Work out the finished part from the listing and answer in its coordinate system (mm). Give positions to 0.01 mm unless a question says otherwise; leave off trailing zeros. Loops run counter-clockwise (first coordinate to the right, second up) from the corner with the lowest first, then second, coordinate; pieces in that order, holes last. Notation, with made-up numbers: (86, 52.25) - (122, 52.25) arc R31 cw to (122, 76.25) - close; hole circle Ø1 at (2, -25). An arc over 180 degrees is marked (long way). One line per question, with ' | ' between items.
from build123d import *

# Parameters (mm, degrees)
SKETCH_1_R          = 1.575
SKETCH_1_R_2        = 14.5
EXTRUDE_1_DEPTH     = 3
CUT_EXTRUDE_START   = -3
CUT_EXTRUDE_1_DEPTH = 3
SKETCH_3_W          = 9
SKETCH_3_H          = 4
EXTRUDE_2_DEPTH     = 3
SKETCH_4_R          = 4
SKETCH_4_R_2        = 1.4
EXTRUDE_3_DEPTH     = 3
SKETCH_5_W          = 57.078231857
SKETCH_5_H          = 48.607322339
CUT_EXTRUDE_2_DEPTH = 10
SKETCH_6_W          = 9
SKETCH_6_H          = 3
EXTRUDE_4_DEPTH     = 3
FILLET_1_R          = 2
FILLET_2_R          = 3
FILLET_3_R          = 2


with BuildPart() as part:
    # 草图1 → 凸台-拉伸1 (new body)
    with BuildSketch(Plane.XY):
        with BuildLine():
            ThreePointArc((7.5, 0), (7.485279444, 0.469671844), (7.441175562, 0.9375))
            Line((7.441175562, 0.9375), (4.960783708, 20.625))
            ThreePointArc((4.960783708, 20.625), (0, 25), (-4.960783708, 20.625))
            Line((-4.960783708, 20.625), (-7.441175562, 0.9375))
            ThreePointArc((-7.441175562, 0.9375), (-7.485279444, 0.469671844), (-7.5, 0))
            Line((-7.5, 0), (-7.5, -69.31788212))
            ThreePointArc((-7.5, -69.31788212), (0, -112), (7.5, -69.31788212))
            Line((7.5, -69.31788212), (7.5, 0))
        make_face()
        with Locations((-12.374368671, -102.374368671)):
            Circle(SKETCH_1_R, mode=Mode.SUBTRACT)
        with Locations((-12.374368671, -77.625631329)):
            Circle(SKETCH_1_R, mode=Mode.SUBTRACT)
        with Locations((0, -90)):
            Circle(SKETCH_1_R_2, mode=Mode.SUBTRACT)
        with Locations((12.374368671, -102.374368671)):
            Circle(SKETCH_1_R, mode=Mode.SUBTRACT)
        with Locations((12.374368671, -77.625631329)):
            Circle(SKETCH_1_R, mode=Mode.SUBTRACT)
        Circle(SKETCH_1_R, mode=Mode.SUBTRACT)
        with Locations((0, 20)):
            Circle(SKETCH_1_R, mode=Mode.SUBTRACT)
    extrude(amount=EXTRUDE_1_DEPTH)

    # 草图2 → 切除-拉伸1 (cut)
    with BuildSketch(Plane.XY.offset(3).offset(CUT_EXTRUDE_START)):
        with BuildLine():
            Line((0, -68), (0, -5))
            ThreePointArc((0, -5), (-2.655442773, -4.236581603), (-4.5, -2.179449472))
            Line((-4.5, -2.179449472), (-4.5, -68.465144533))
            ThreePointArc((-4.5, -68.465144533), (-2.261988032, -68.116595097), (0, -68))
        make_face()
        with BuildLine():
            ThreePointArc((4.5, -2.179449472), (2.655442773, -4.236581603), (0, -5))
            Line((0, -5), (0, -68))
            ThreePointArc((0, -68), (2.261988032, -68.116595097), (4.5, -68.465144533))
            Line((4.5, -68.465144533), (4.5, -2.179449472))
        make_face()
        with BuildLine():
            Line((-2.557135445, 15.70336663), (-4.192274153, 2.724855487))
            ThreePointArc((-4.192274153, 2.724855487), (0, 5), (4.192274153, 2.724855487))
            Line((4.192274153, 2.724855487), (2.557135445, 15.70336663))
            ThreePointArc((2.557135445, 15.70336663), (0, 15), (-2.557135445, 15.70336663))
        make_face()
    extrude(amount=CUT_EXTRUDE_1_DEPTH, mode=Mode.SUBTRACT)

    # 草图3 → 凸台-拉伸2 (add)
    with BuildSketch(Plane.XY.offset(3)):
        with Locations((0, -45)):
            Rectangle(SKETCH_3_W, SKETCH_3_H)
        with Locations((0, -25)):
            Rectangle(SKETCH_3_W, SKETCH_3_H)
    extrude(amount=-EXTRUDE_2_DEPTH)

    # 草图4 → 凸台-拉伸3 (add)
    # profile 1 of 2: a face of its own
    with BuildSketch(Plane.XY.offset(3)):
        with Locations((-9, -61.2)):
            Circle(SKETCH_4_R)
        with Locations((-9, -61.2)):
            Circle(SKETCH_4_R_2, mode=Mode.SUBTRACT)
    # profile 2 of 2: a face of its own
    with BuildSketch(Plane.XY.offset(3)):
        with Locations((9, -61.2)):
            Circle(SKETCH_4_R)
        with Locations((9, -61.2)):
            Circle(SKETCH_4_R_2, mode=Mode.SUBTRACT)
    extrude(amount=-EXTRUDE_3_DEPTH)

    # 草图5 → 切除-拉伸2 (cut)
    with BuildSketch(Plane.XY.offset(3)):
        with Locations((3.178219729, -91.30366117)):
            Rectangle(SKETCH_5_W, SKETCH_5_H)
    extrude(amount=-CUT_EXTRUDE_2_DEPTH, mode=Mode.SUBTRACT)

    # 草图6 → 凸台-拉伸4 (add)
    with BuildSketch(Plane.XY.offset(3)):
        with Locations((0, -65.5)):
            Rectangle(SKETCH_6_W, SKETCH_6_H)
    extrude(amount=-EXTRUDE_4_DEPTH)

    # 圆角1
    fillet_1_edges = [part.edges().sort_by_distance(p)[0] for p in [
        (-4.5, -27, 1.5),
        (-4.5, -23, 1.5),
        (4.5, -23, 1.5),
        (4.5, -27, 1.5),
        (-2.557135445, 15.70336663, 1.5),
        (2.557135445, 15.70336663, 1.5),
        (4.192274153, 2.724855487, 1.5),
        (-4.192274153, 2.724855487, 1.5),
        (-4.5, -2.179449472, 1.5),
        (4.5, -2.179449472, 1.5),
        (-4.5, -47, 1.5),
        (-4.5, -43, 1.5),
        (4.5, -43, 1.5),
        (4.5, -47, 1.5),
    ]]
    fillet(fillet_1_edges, radius=FILLET_1_R)

    # 圆角2
    # the kernel refuses this fillet: 3 mm, written as the material it adds along each edge
    with BuildSketch(Plane(origin=(-7.5, -64.908099244, 0), x_dir=(0, -1, 0), z_dir=(0, 0, 1))) as fillet_2_piece_1:
        with BuildLine():
            CenterArc((3.170220896, -2.799504541), FILLET_2_R, 111.06581136, 58.235536144)
            Line((0.222369408, -2.242574024), (0.163412378, -2.231435413))
            ThreePointArc((0.163412378, -2.231435413), (0.21267274, -1.11122365), (-0.055621489, -0.0225))
            Line((-0.055621489, -0.0225), (0, 0.06))
            ThreePointArc((0, 0.06), (1.045950378, 0.06), (2.070334354, 0.055990091))
            Line((2.070334354, 0.055990091), (2.091900756, 0))
        make_face()
    extrude(amount=3)
    with BuildSketch(Plane(origin=(-7.5, -57.491900756, 0), x_dir=(0, 1, 0), z_dir=(0, 0, 1))) as fillet_2_piece_2:
        with BuildLine():
            CenterArc((3.129297922, 3), FILLET_2_R, 192.373625116, 77.626374884)
            Line((0.198984851, 2.357142857), (0.14037859, 2.344285714))
            ThreePointArc((0.14037859, 2.344285714), (0.217936404, 1.168572647), (-0.055621489, 0.0225))
            Line((-0.055621489, 0.0225), (0, -0.06))
            Line((0, -0.06), (3.129297922, -0.06))
            Line((3.129297922, -0.06), (3.129297922, 0))
        make_face()
    extrude(amount=3)
    with BuildSketch(Plane(origin=(7.5, -64.908099244, 0), x_dir=(0, -1, 0), z_dir=(0, 0, 1))) as fillet_2_piece_3:
        with BuildLine():
            CenterArc((3.170220896, 2.799504541), FILLET_2_R, 190.698652496, 58.235536144)
            Line((0.222369408, 2.242574024), (0.163412378, 2.231435413))
            ThreePointArc((0.163412378, 2.231435413), (0.21267274, 1.11122365), (-0.055621489, 0.0225))
            Line((-0.055621489, 0.0225), (0, -0.06))
            ThreePointArc((0, -0.06), (1.045950378, -0.06), (2.070334354, -0.055990091))
            Line((2.070334354, -0.055990091), (2.091900756, 0))
        make_face()
    extrude(amount=3)
    with BuildSketch(Plane(origin=(7.5, -57.491900756, 0), x_dir=(0.996455748224994, 0.08411861761445558, 0), z_dir=(0, 0, 1))) as fillet_2_piece_4:
        with BuildLine():
            CenterArc((3.25259946, 2.865851049), FILLET_2_R, 175.17465614, 77.626374884)
            Line((0.263232215, 3.118206902), (0.20344487, 3.123254019))
            Line((0.20344487, 3.123254019), (-0.059787345, 0.005047117))
            Line((-0.059787345, 0.005047117), (0.017741452, -0.057317021))
            ThreePointArc((0.017741452, -0.057317021), (1.18276344, 0.118865267), (2.347785428, -0.057317021))
            Line((2.347785428, -0.057317021), (2.36552688, 0))
        make_face()
    extrude(amount=3)

    # 圆角3
    fillet_3_edges = [part.edges().sort_by_distance(p)[0] for p in [
        (-7.5, -67, 1.5),
        (7.5, -67, 1.5),
        (-4.5, -64, 1.5),
        (4.5, -64, 1.5),
    ]]
    fillet(fillet_3_edges, radius=FILLET_3_R)


solid = part.part
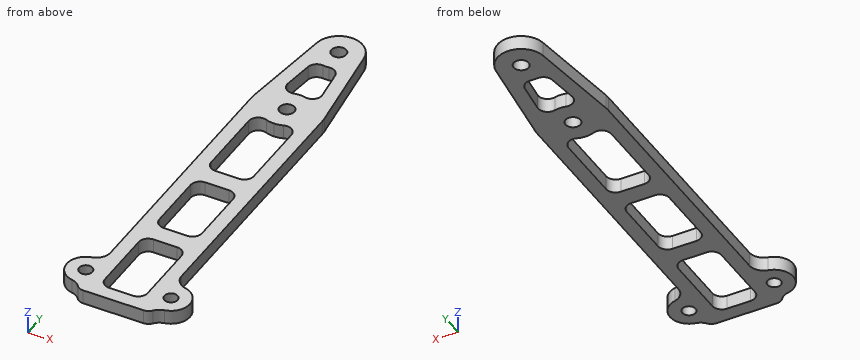
1. Consider L1, parallel to X at y = -50.5, z = 2.3; L2, parallel to Y at x = -7.75, z = 2.8; L3, parallel to X at y = -59.5, z = 2.65. Determine where each line is inside the solid, lowest interval first.
Evaluation:
L1: -7.5 to -4.5, 4.5 to 7.5 | L2: -66.44 to -61.83, -60.57 to -55.56 | L3: -12.62 to -4.5, 4.5 to 12.62
2. Find section A-A on y = -61.2. Write down the section's boundary in (x, z), then the cut area to 3 significant figures.
Evaluation:
outline: (-13, 0) - (-10.4, 0) - (-10.4, 3) - (-13, 3) - close; (-7.6, 0) - (-4.5, 0) - (-4.5, 3) - (-7.6, 3) - close; (4.5, 0) - (7.6, 0) - (7.6, 3) - (4.5, 3) - close; (10.4, 0) - (13, 0) - (13, 3) - (10.4, 3) - close | area: 34.2 mm2
3. Flat-ended cylindrical pins translate along their axes: pin 1 (1.5 mm diameter, centred on y = -32.5, z = 2, fed in from -X); pin 2 (0.9 mm diameter, centred on y = -25.5, z = 1.5, fed in from +X). Find the tip coordinate at first contact, or state that the pin passes through.
Evaluation:
pin 1: x = -7.5 | pin 2: x = 7.5
4. Find section B-B on y = -8. Write down the section's boundary in (x, z), then the cut area to 3 significant figures.
Evaluation:
outline: (-7.5, 0) - (-4.5, 0) - (-4.5, 3) - (-7.5, 3) - close; (4.5, 0) - (7.5, 0) - (7.5, 3) - (4.5, 3) - close | area: 18.0 mm2
5. Find section D-D on y = -28. Write down the section's boundary in (x, z), then the cut area to 3 significant figures.
Evaluation:
outline: (-7.5, 0) - (-4.23, 0) - (-4.23, 3) - (-7.5, 3) - close; (4.23, 0) - (7.5, 0) - (7.5, 3) - (4.23, 3) - close | area: 19.6 mm2
6. Find section C-C on z = 1.6. State how many separate pieces and enclosed holes the cut face has, then the cut area to 3 significant figures.
Evaluation:
separate pieces: 1 | enclosed holes: 8 | area: 833 mm2
